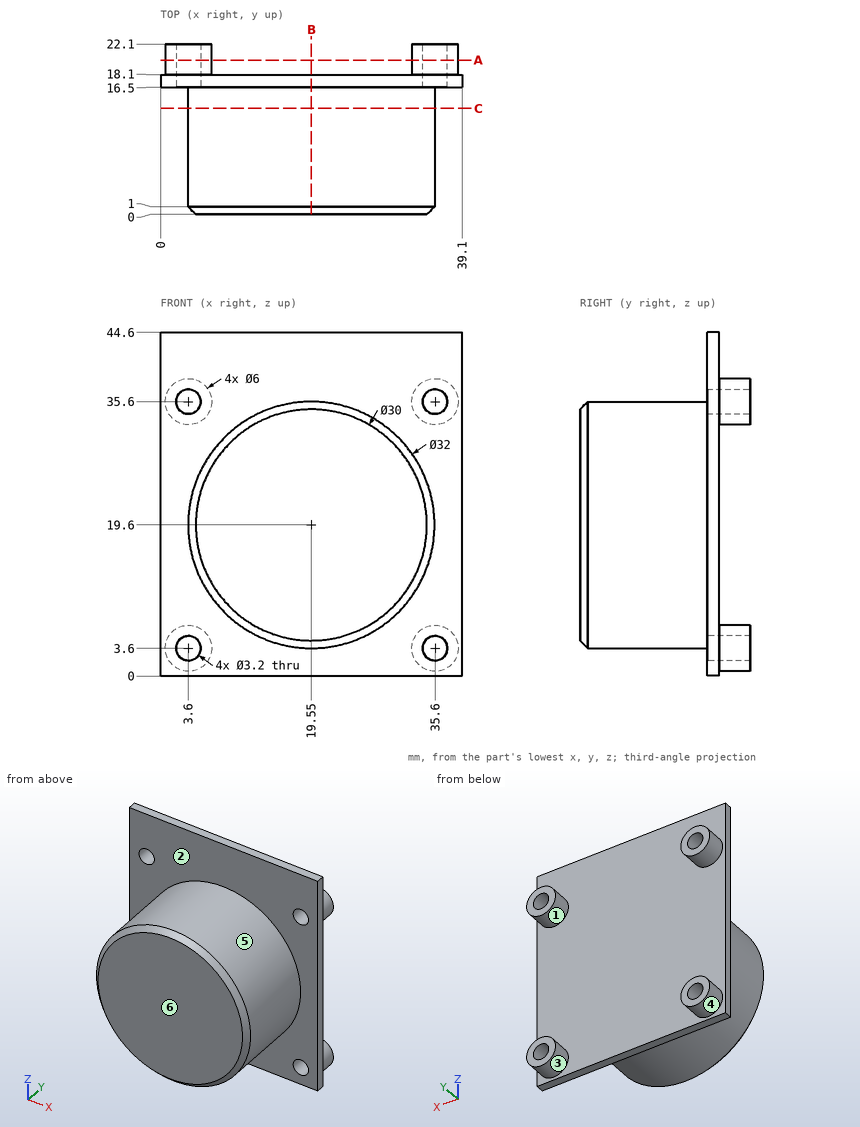
The drawing under review shows one solid part. Ordinate dimensions are in mm from its lowest x, y, z. A direction names the side the tool comes from. Give positions to 0.01 mm unless a question says otherwise; leave off trailing zeros. Loops run counter-clockwise (first coordinate to the right, second up) from the corner with the lowest first, then second, coordinate; pieces in that order, holes last. Notation, with made-up numbers: M 8.5,-11 L 60.5,-11 A5 cw 60.5,-4 Z; hole C -9,-30 d11. An arc over 180 degrees is marked long. One line per item, written item: value. Start each with the question number.
Q1. Draft analysis for pull direction X (two halves, no side actions). For the marked faces 3, 4, 5 and 6, state which applies: released by +X, released by -X, zero draft, split by the parting line, or undercut.
Q2. For L1, parallel to X at y = 20.95, z = 3.6; L2, parallel to X at y = 17.65, z = 3.6, list the stretches that pass through material, from the lowest coordinate up.
Q3. Add section C-C (y = 13.75). Give the boundary of the cut face in (x, z), and give its area (3 significant figures).
Q4. Machinability: for the marked faces 1 and 2, which of the approach directions +Z, -Z, +X, -X, +Y, -Y give a long, thin tool a straight path to every point of the face, cutting with its end or side? Answer none if there is none.
Q5. Add section B-B (x = 19.55). Give the boundary of the cut face in (y, z), and give its area (3 significant figures).
Q6. Add section A-A (y = 20). Give the boundary of the cut face in (x, z), and give its area (3 significant figures).
Q7. Clearance check with flat-ended pins moving along their axes: pin 1 Ø5 at (y, z) = (5, 8) entering from -X; pin 2 Ø1.5 at (x, z) = (8, 8) entering from +Y; pin 3 Ø1 at (x, y) = (18.5, 6.5) entering from +Z. State where each tip first meets the part, or that it passes through.
Reply:
1. face 3: undercut
1. face 4: undercut
1. face 5: split by the parting line
1. face 6: zero draft
2. L1: 0.6 to 2, 5.2 to 6.6, 32.6 to 34, 37.2 to 38.6
2. L2: 0 to 2, 5.2 to 34, 37.2 to 39.1
3. outline: C 19.55,19.6 d32
3. area: 804 mm²
4. face 1: +Y
4. face 2: -Y
5. outline: M 0,4.6 L 1,3.6 L 16.5,3.6 L 16.5,0 L 18.1,0 L 18.1,44.6 L 16.5,44.6 L 16.5,35.6 L 1,35.6 L 0,34.6 Z
5. area: 598 mm²
6. outline: C 3.6,3.6 d6; C 3.6,35.6 d6; C 35.6,3.6 d6; C 35.6,35.6 d6; hole C 3.6,3.6 d3.2; hole C 3.6,35.6 d3.2; hole C 35.6,3.6 d3.2; hole C 35.6,35.6 d3.2
6. area: 80.9 mm²
7. pin 1: x = 6.39
7. pin 2: y = 18.1
7. pin 3: z = 35.59
